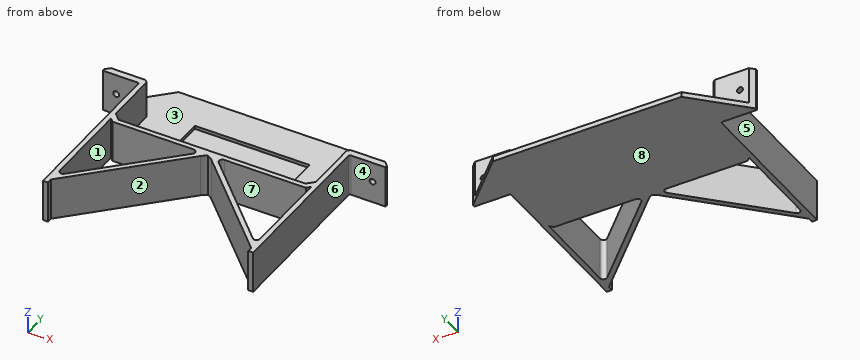
```python
from build123d import *

# Parameters (mm, degrees)
SKETCH1_W            = 125
SKETCH1_H            = 40
BOSS_EXTRUDE1_DEPTH  = 3
SKETCH2_W            = 3
SKETCH2_H            = 40
BOSS_EXTRUDE2_DEPTH  = 22
SKETCH4_W            = 25
SKETCH4_H            = 4
BOSS_EXTRUDE4_DEPTH  = 21.59
SKETCH5_W            = 25
SKETCH5_H            = 4
BOSS_EXTRUDE5_DEPTH  = 21.59
SKETCH6_W            = 168.18
SKETCH6_H            = 25.4
BOSS_EXTRUDE6_DEPTH  = 3
CHAMFER1_SIZE        = 28
SKETCH7_W            = 68.2
SKETCH7_H            = 26
CUT_EXTRUDE1_DEPTH   = 2
SKETCH9_W            = 119
SKETCH9_H            = 3
BOSS_EXTRUDE7_DEPTH  = 22
CHAMFER2_SIZE        = 4
CHAMFER3_SIZE        = 5
SKETCH11_R           = 1.75
CUT_EXTRUDE3_DEPTH   = 5
FILLET1_R            = 1
CHAMFER4_SIZE        = 1.5
BOSS_EXTRUDE10_DEPTH = 25
FILLET2_R            = 10
FILLET3_R            = 2
FILLET4_R            = 2


with BuildPart() as part:
    # Sketch1 → Boss-Extrude1 (new body)
    with BuildSketch(Plane.XY):
        Rectangle(SKETCH1_W, SKETCH1_H)
    extrude(amount=BOSS_EXTRUDE1_DEPTH)

    # Sketch2 → Boss-Extrude2 (add)
    with BuildSketch(Plane.XY.offset(3)):
        with Locations((-61, 0)):
            Rectangle(SKETCH2_W, SKETCH2_H)
        with Locations((61, 0)):
            Rectangle(SKETCH2_W, SKETCH2_H)
    extrude(amount=BOSS_EXTRUDE2_DEPTH)

    # Sketch4 → Boss-Extrude4 (add)
    with BuildSketch(Plane.ZY.offset(62.5)):
        with Locations((12.5, 18)):
            Rectangle(SKETCH4_W, SKETCH4_H)
    extrude(amount=BOSS_EXTRUDE4_DEPTH)

    # Sketch5 → Boss-Extrude5 (add)
    with BuildSketch(Plane(origin=(62.5, 0, 0), x_dir=(0, 0, -1), z_dir=(1, 0, 0))):
        with Locations((-12.5, 18)):
            Rectangle(SKETCH5_W, SKETCH5_H)
    extrude(amount=BOSS_EXTRUDE5_DEPTH)

    # Sketch6 → Boss-Extrude6 (add)
    with BuildSketch(Plane(origin=(0, 0, 0), x_dir=(-1, 0, 0), z_dir=(0, 0, -1))):
        with Locations((0, 32.7)):
            Rectangle(SKETCH6_W, SKETCH6_H)
    extrude(amount=-BOSS_EXTRUDE6_DEPTH)

    # Chamfer1
    chamfer1_edges = [part.edges().sort_by_distance(p)[0] for p in [
        (-84.09, 45.4, 1.5),
        (84.09, 45.4, 1.5),
    ]]
    chamfer(chamfer1_edges, length=CHAMFER1_SIZE)

    # Sketch7 → Cut-Extrude1 (cut)
    with BuildSketch(Plane.XY.offset(3)):
        with Locations((0, 11.217156681)):
            Rectangle(SKETCH7_W, SKETCH7_H)
    extrude(amount=-CUT_EXTRUDE1_DEPTH, mode=Mode.SUBTRACT)

    # Sketch9 → Boss-Extrude7 (add)
    with BuildSketch(Plane.XY.offset(3)):
        with Locations((0, -18.5)):
            Rectangle(SKETCH9_W, SKETCH9_H)
    extrude(amount=BOSS_EXTRUDE7_DEPTH)

    # Chamfer2
    chamfer2_edges = [part.edges().sort_by_distance(p)[0] for p in [
        (-59.5, -17, 14),
        (59.5, -17, 14),
    ]]
    chamfer(chamfer2_edges, length=CHAMFER2_SIZE)

    # Chamfer3
    chamfer3_edges = [part.edges().sort_by_distance(p)[0] for p in [
        (62.5, -20, 12.5),
        (-62.5, -20, 12.5),
    ]]
    chamfer(chamfer3_edges, length=CHAMFER3_SIZE)

    # Sketch11 → Cut-Extrude3 (cut)
    with BuildSketch(Plane(origin=(0, 20, 0), x_dir=(1, 0, 0), z_dir=(0, 1, 0))):
        with Locations(Location((-76.11, -13, 0), (0, 0, 270))):
            Circle(SKETCH11_R)
        with Locations(Location((76.29, -13, 0), (0, 0, 270))):
            Circle(SKETCH11_R)
    extrude(amount=-CUT_EXTRUDE3_DEPTH, mode=Mode.SUBTRACT)

    # Fillet1
    fillet1_edges = [part.edges().sort_by_distance(p)[0] for p in [
        (-62.5, 16, 12.5),
        (62.5, 16, 12.5),
    ]]
    fillet(fillet1_edges, radius=FILLET1_R)

    # Chamfer4
    chamfer4_edges = [part.edges().sort_by_distance(p)[0] for p in [
        (-59.5, 20, 14),
        (59.5, 20, 14),
    ]]
    chamfer(chamfer4_edges, length=CHAMFER4_SIZE)

    # Sketch12 → Boss-Extrude10 (add)
    with BuildSketch(Plane.XY.offset(25)):
        Polygon((-0.275787659, -20.275787659), (-59.5, -79.5), (-59.5, -82.5), (-62.5, -82.5), (-62.5, -15), (-59.5, -15), (-59.5, -75.257359313), (-4.242640687, -20), (0, -20), (4.242640687, -20), (59.5, -75.257359313), (59.5, -15), (62.5, -15), (62.5, -82.5), (59.5, -82.5), (59.5, -79.5), (0.275787659, -20.275787659), align=None)
    extrude(amount=-BOSS_EXTRUDE10_DEPTH)

    # Fillet2
    # the kernel refuses this fillet: 10 mm, written as the material it adds along each edge
    with BuildSketch(Plane(origin=(0.275787659, -20.275787659, 25), x_dir=(0.7071067811865169, -0.7071067811865782, 0), z_dir=(0, 0, -1)), Plane(origin=(-0.275787659, -20.275787659, 25), x_dir=(1, 0, 0), z_dir=(0, 0, -1))) as fillet2_piece_1:
        with BuildLine():
            CenterArc((FILLET2_R * 0.414213562373, FILLET2_R), FILLET2_R, 225, 45)
            Line((-FILLET2_R * 0.292893218813, FILLET2_R * 0.292893218813), (0, 0))
            Line((0, 0), (FILLET2_R * 0.414213562373, 0))
        make_face()
    extrude(amount=25)

    # Fillet3
    fillet3_edges = [part.edges().sort_by_distance(p)[0] for p in [
        (59.5, -75.257359313, 12.5),
        (-59.5, -75.257359313, 12.5),
    ]]
    fillet(fillet3_edges, radius=FILLET3_R)

    # Fillet4
    fillet4_edges = [part.edges().sort_by_distance(p)[0] for p in [
        (-4.242640687, -20, 12.5),
        (4.242640687, -20, 12.5),
    ]]
    fillet(fillet4_edges, radius=FILLET4_R)


solid = part.part
```
Design review of the part built by this model. Coordinates are the model's own, in mm. Face numbers are marked on the shaded views. A direction names the side the tool comes from. Coordinates: 2 decimals unless noted, no trailing zeros. Order: outer loops, then holes, each group sorted by start corner. A loop starts at its lowest first (then second) coordinate and runs counter-clockwise, first axis right, second up.
1) Take a section at B-B, the plane y = -52. Give the boundary of the cut face in (x, z), and give its area (3 significant figures).
2) Mouldability with a two-part tool opening along X and no side actions: class the marked faces 5, 6, 7 and 8 as +X half, -X half, draft (parallel to the pull), parting line (faces both ways), or undercut.
3) For the marked faces 1, 2, 3 and 4, list the 3-axis set-ups (+Z, -Z, +X, -X, +Y, -Y) from which the entire face can be reached by the end or side of a thin tool; tool diameter is ignored.
4) Clearance check with flat-ended pins moving along their axes: pin 1 (1 mm diameter, centred on x = 32, z = 13, fed in from +Y); pin 2 (10 mm diameter, centred on x = 35.5, y = 4.5, fed in from -Z); pin 3 (2 mm diameter, centred on y = 5.5, z = 2, fed in from -X); pin 4 (7.5 mm diameter, centred on x = 28.5, z = 7, fed in from -Y). State where each tip first meets the part, or that it passes through.
5) Take a section at C-C, the plane z = 13. State how many separate pieces and enclosed holes the cut face has, and give its area (3 significant figures).
6) Take a section at D-D, the plane x = -76.11. Give the boundary of the cut face in (y, z).
7) Take a section at A-A, the plane x = 76.29. Give the boundary of the cut face in (y, z).
8) Wall thickness on line 1 along X through (y, z) = (17.15, 13); line 2 along Z through (x, y) = (-76.11, 17.8); line 3 along X through (y, z) = (18.15, 13): over which ranges is each line inside the solid? List them lowest first.
Returned:
1. outline: (-62.5, 0) - (-59.5, 0) - (-59.5, 25) - (-62.5, 25) - close; (-36.24, 0) - (-32, 0) - (-32, 25) - (-36.24, 25) - close; (32, 0) - (36.24, 0) - (36.24, 25) - (32, 25) - close; (59.5, 0) - (62.5, 0) - (62.5, 25) - (59.5, 25) - close
1. area: 362 mm2
2. face 5: -X half
2. face 6: +X half
2. face 7: undercut
2. face 8: draft
3. face 1: +Z, -Z
3. face 2: +Z, -Z, -Y
3. face 3: +Z, +Y
3. face 4: +Z, -Z, +X, -Y
4. pin 1: stops at y = -17
4. pin 2: stops at z = 0
4. pin 3: stops at x = -62.5
4. pin 4: stops at y = -52.25
5. separate pieces: 3
5. enclosed holes: 2
5. area: 1,630 mm2
6. outline: (16, 0) - (25.38, 0) - (25.38, 3) - (20, 3) - (20, 11.25) - (16, 11.25) - close; (16, 14.75) - (20, 14.75) - (20, 25) - (16, 25) - close
7. outline: (16, 0) - (25.2, 0) - (25.2, 3) - (20, 3) - (20, 11.25) - (16, 11.25) - close; (16, 14.75) - (20, 14.75) - (20, 25) - (16, 25) - close
8. line 1: x = -84.09 to -77.86, -74.36 to -59.5, 59.5 to 74.54, 78.04 to 84.09
8. line 2: z = 0 to 11.25, 14.75 to 25
8. line 3: x = -83.34 to -77.86, -74.36 to -59.5, 59.5 to 74.54, 78.04 to 83.34
